Autodesk Inventor part; units mm, degrees
ref_plane "YZ Plane" through (0, 0, 0) normal (1, 0, 0) x (0, 1, 0)
ref_plane "XZ Plane" through (0, 0, 0) normal (0, 1, 0) x (-1, 0, 0)
ref_plane "XY Plane" through (0, 0, 0) normal (0, 0, 1) x (1, 0, 0)
sketch "Boceto1" plane through (0, 0, 0) normal (0, 1, 0) x (-1, 0, 0)
  circle A0 centre (0, 0) radius 4.5
  dimension "d0" = 9
extrude "Extrusión1" add sketch "Boceto1" along normal blind 1.6
sketch "Boceto2" plane through (0, 1.6, 0) normal (0, 1, 0) x (1, 0, 0)
  circle A0 centre (0, 0) radius 2.5
  dimension "d3" = 5
extrude "Extrusión2" add sketch "Boceto2" along normal blind 50
fillet "Empalme1" radius 0.4 1 edges at (4.5, 0, 0)
fillet "Empalme2" radius 0.2 1 edges at (4.5, 1.6, 0)
sketch "Boceto3" plane through (0, 0, 0) normal (0, -1, 0) x (1, 0, 0)
  line L0 (-1.7321, 0) -> (-0.866, 1.5)
  line L1 (-0.866, 1.5) -> (0.866, 1.5)
  line L2 (0.866, 1.5) -> (1.7321, 0)
  line L3 (1.7321, 0) -> (0.866, -1.5)
  line L4 (0.866, -1.5) -> (-0.866, -1.5)
  line L5 (-0.866, -1.5) -> (-1.7321, 0)
  point P0 (0, 0)
  point P1 (0, 0)
  dimension "d8" = 3
extrude "Extrusión3" cut sketch "Boceto3" against normal blind 2.5
chamfer "Chaflán1" distance 0.5 angle 45 1 edges at (-2.5, 51.6, 0)
thread "Rosca2"
properties part number "Perno M5x8 cabeza plana" material "Hierro, gris"
Source: CAD feature listing. Evaluate the final solid. Frame: model axes, mm. A direction names the side the tool comes from. Coordinates: 2 decimals unless noted, no trailing zeros. Order: outer loops, then holes, each group sorted by start corner. A loop starts at its lowest first (then second) coordinate and runs counter-clockwise, first axis right, second up. Notation, with made-up numbers: (35, 33.5) - (93, 33.5) arc R3 ccw to (93, 38.5) - close; hole circle Ø6 at (27.5, -36.5). An arc over 180 degrees is marked (long way). One line per item, written item: value.
1) Cut plane B-B on y = 11.5. Output: boundary loops of the cut face in (x, z).
Computed values:
outline: circle Ø5 at (0, 0)
2) Mould query, pull axis X, two halves, no side actions, for faces 1 (the face through (0, 51.6, 0)), 2 (the face through (1.293, 1.232, 0.76)), 3 (the face through (0.59, 0.89, -4.46)). Classes: released by +X, released by -X, zero draft, split by the parting line, or undercut.
Computed values:
face 1: zero draft
face 2: undercut
face 3: split by the parting line
3) Contact query for flat-ended pins moving along their axis: pin 1 (1 mm diameter, centred on y = 20, z = 0.5, fed in from -X); pin 2 (1 mm diameter, centred on x = 2.5, y = 38.5, fed in from +Z); pin 3 (1.5 mm diameter, centred on y = 17.5, z = -1.5, fed in from +X). Output: stop coordinate, or through.
Computed values:
pin 1: stops at x = -2.5
pin 2: stops at z = 1.5
pin 3: stops at x = 2.38
4) Cut plane A-A on x = 0. Output: boundary loops of the cut face in (y, z), plus the area to 3 significant figures.
Computed values:
outline: (0, -4.1) arc R0.4 ccw to (0.4, -4.5) - (1.4, -4.5) arc R0.2 ccw to (1.6, -4.3) - (1.6, -2.5) - (51.1, -2.5) - (51.6, -2) - (51.6, 2) - (51.1, 2.5) - (1.6, 2.5) - (1.6, 4.3) arc R0.2 ccw to (1.4, 4.5) - (0.4, 4.5) arc R0.4 ccw to (0, 4.1) - (0, 1.5) - (2.5, 1.5) - (2.5, -1.5) - (0, -1.5) - close
area: 257 mm^2
5) Reachability of faces 4 (the face through (0, 0, -2)), 5 (the face through (-2, 1.6, -2)), 6 (the face through (0, 1, 1.5)) from +Z, -Z, +X, -X, +Y, -Y: full face, straight path, thin tool, end or side. Return the list, or none.
Computed values:
face 4: +Z, -Z, +X, -X, -Y
face 5: +Y
face 6: -Y
6) Ray query, line 1 (Z direction, x = 0, y = 31); line 2 (Y direction, x = -3.25, z = -2.25); line 3 (Z direction, x = -2, y = 27). Return the intervals inside material, ascending. Write a range as [from, to].
Computed values:
line 1: z = [-2.5, 2.5]
line 2: y = [0, 1.6]
line 3: z = [-1.5, 1.5]
